Check sheet for the drawn part. Datum: minimum x, y, z corner. Units: mm. A direction names the side the tool comes from. Give positions to 0.01 mm unless a question says otherwise; leave off trailing zeros. Loops run counter-clockwise (first coordinate to the right, second up) from the corner with the lowest first, then second, coordinate; pieces in that order, holes last.
1. Cross-section at C-C, the plane x = 13.75. Record the cut outline in (y, z).
2. Release check for a two-part mould opening along X. For the marked faces 3, 4, 5 and 6 record: +X half, -X half, draft (parallel to the pull), parting line (faces both ways), or undercut.
3. Material ranges on L1, parallel to X at y = 4.75, z = 3.25; L2, parallel to Y at x = 12, z = 2.25; L3, parallel to X at y = 9.25, z = 5.5, recorded low to high.
4. Tool access check on the marked faces 1 and 2. Record the directions out of +Z, -Z, +X, -X, +Y, -Y that give a thin tool (end or side, any length) a straight path to the whole face; none if there is none.
5. Go/stop test with flat-tipped pins: pin 1 Ø1.5 at (y, z) = (13, 1) entering from +X; pin 2 Ø1 at (y, z) = (12, 4) entering from -X; pin 3 Ø3.5 at (x, z) = (2.5, 3) entering from -Y (1 decimal). Record where each tip stops, or that it passes through.
6. Cross-section at B-B, the plane z = 4.5. Record the cut outline in (x, y) (1 decimal).
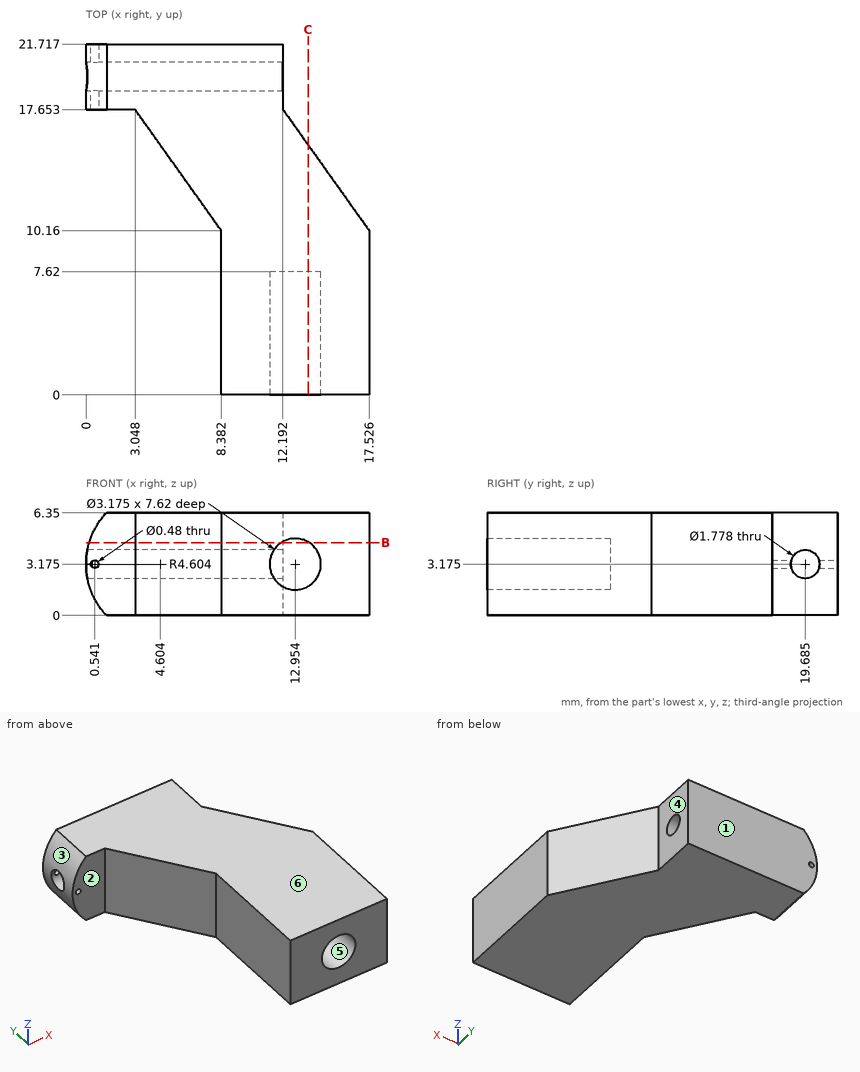
Result:
1. outline: (0, 0) - (15.46, 0) - (15.46, 6.35) - (0, 6.35) - (0, 4.55) - (7.62, 4.55) - (7.62, 1.8) - (0, 1.8) - close
2. face 3: -X half
2. face 4: +X half
2. face 5: undercut
2. face 6: draft
3. L1: x = 8.38 to 11.37, 14.54 to 17.53
3. L2: y = 7.62 to 21.72
3. L3: x = 8.38 to 17.53
4. face 1: +Z, -Z, +X, -X, +Y
4. face 2: +Z, -Z, -X, -Y
5. pin 1: stops at x = 16.04
5. pin 2: stops at x = 6.72
5. pin 3: stops at y = 16
6. outline: (0.2, 17.7) - (3, 17.7) - (8.4, 10.2) - (8.4, 0) - (12.1, 0) - (12.1, 7.6) - (13.8, 7.6) - (13.8, 0) - (17.5, 0) - (17.5, 10.2) - (12.2, 17.7) - (12.2, 21.7) - (0.2, 21.7) - close
